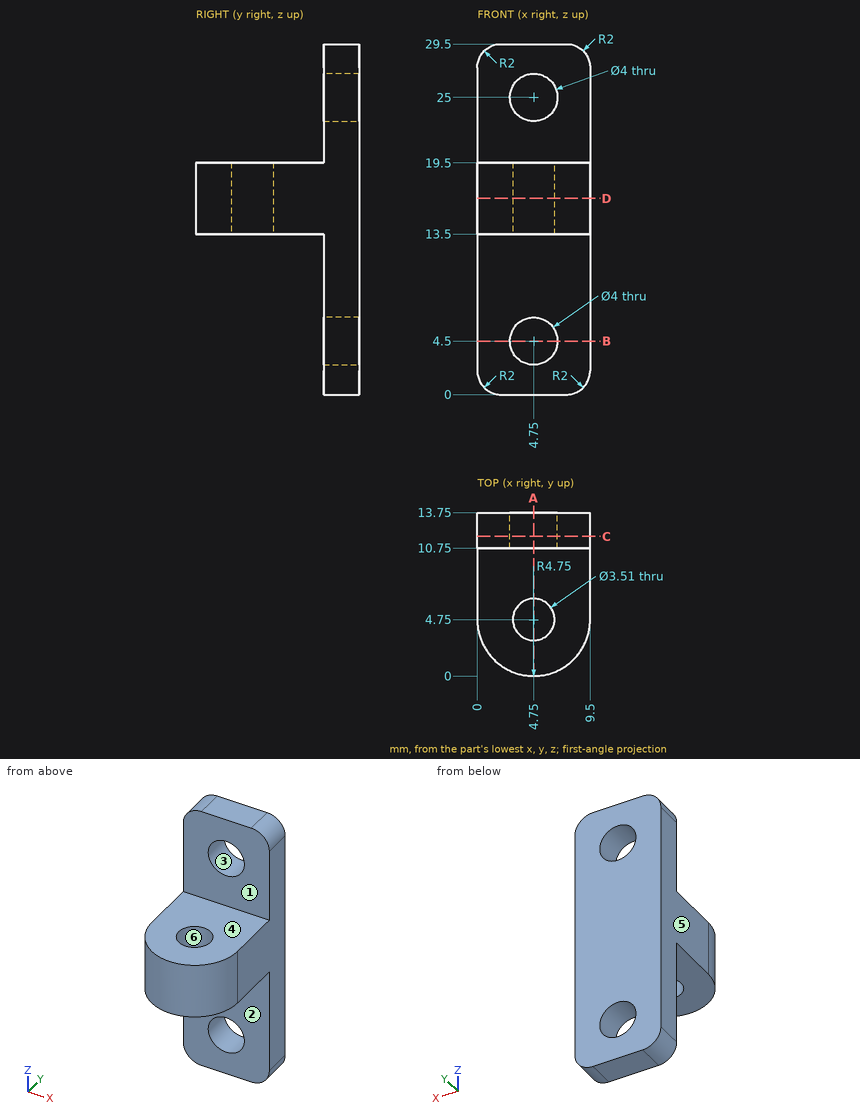
Job drawing, mm, ordinate dimensions from the low corner. One solid piece. A direction names the side the tool comes from. Give positions to 0.01 mm unless a question says otherwise; leave off trailing zeros. Loops run counter-clockwise (first coordinate to the right, second up) from the corner with the lowest first, then second, coordinate; pieces in that order, holes last. Notation, with made-up numbers: M -33.75,85.25 L 2.25,85.25 A24 cw 2.25,108.25 Z; hole C 60.5,-12 d9. An arc over 180 degrees is marked long. Return JSON: item names as keys, results as strings.
1) Flat gauge pins, fed straight in: pin 1 Ø3 at (x, z) = (6.5, 24) entering from -Y; pin 2 Ø5 at (x, y) = (3, 8) entering from -Z; pin 3 Ø3 at (x, y) = (3.5, 5.5) entering from +Z; pin 4 Ø1.5 at (x, y) = (5.5, 10.5) entering from -Z. Where does each tip first touch, or does it go through?
Calculated:
{"pin 1": "stops at y = 10.75", "pin 2": "stops at z = 13.5", "pin 3": "stops at z = 19.5", "pin 4": "stops at z = 0"}
2) Saw through at D-D, the plane z = 16.5. List the corners of the cut face in (x, y) (3 decimals), then the cut area to 3 significant figures.
Calculated:
{"outline": "M 0,4.75 A4.75 ccw 9.5,4.75 L 9.5,13.75 L 0,13.75 Z; hole C 4.75,4.75 d3.51", "area": "111 mm2"}
3) Saw through at C-C, the plane y = 11.75. List the corners of the cut face in (x, z), then the cut area to 3 significant figures.
Calculated:
{"outline": "M 0,2 A2 ccw 2,0 L 7.5,0 A2 ccw 9.5,2 L 9.5,27.5 A2 ccw 7.5,29.5 L 2,29.5 A2 ccw 0,27.5 Z; hole C 4.75,4.5 d4; hole C 4.75,25 d4", "area": "252 mm2"}
4) Drill centre lines: line 1 (Y direction, x = 4.75, z = 18.1) (3 decimals); line 2 (X direction, y = 13, z = 4.5); line 3 (Y direction, x = 1.25, z = 6). Where is each one in solid material? Low to high.
Calculated:
{"line 1": "y = 0 to 2.995, 6.505 to 13.75", "line 2": "x = 0 to 2.75, 6.75 to 9.5", "line 3": "y = 10.75 to 13.75"}
5) Pull direction X, two halves, no side cores. Call the marked faces 4, 5 and 6: released by +X, released by -X, zero draft, split by the parting line, or undercut.
Calculated:
{"face 4": "zero draft", "face 5": "released by -X", "face 6": "undercut"}
6) Saw through at B-B, the plane z = 4.5. List the corners of the cut face in (x, y), then the cut area to 3 significant figures.
Calculated:
{"outline": "M 0,10.75 L 2.75,10.75 L 2.75,13.75 L 0,13.75 Z; M 6.75,10.75 L 9.5,10.75 L 9.5,13.75 L 6.75,13.75 Z", "area": "16.5 mm2"}
7) 3-axis set-ups, long thin cutter, end or side, ignore diameter. For the marked faces 1, 2 and 3: which of +Z, -Z, +X, -X, +Y, -Y reach the whole face in a straight line?
Calculated:
{"face 1": "+Z, +X, -X, -Y", "face 2": "-Z, +X, -X, -Y", "face 3": "+Y, -Y"}
8) Saw through at A-A, the plane x = 4.75. List the corners of the cut face in (y, z) (3 decimals), then the cut area to 3 significant figures.
Calculated:
{"outline": "M 0,13.5 L 2.995,13.5 L 2.995,19.5 L 0,19.5 Z; M 6.505,13.5 L 10.75,13.5 L 10.75,6.5 L 13.75,6.5 L 13.75,23 L 10.75,23 L 10.75,19.5 L 6.505,19.5 Z; M 10.75,0 L 13.75,0 L 13.75,2.5 L 10.75,2.5 Z; M 10.75,27 L 13.75,27 L 13.75,29.5 L 10.75,29.5 Z", "area": "108 mm2"}
